Autodesk Inventor part; units mm, degrees
ref_plane "YZ Plane" through (0, 0, 0) normal (1, 0, 0) x (0, 1, 0)
ref_plane "XZ Plane" through (0, 0, 0) normal (0, 1, 0) x (-1, 0, 0)
ref_plane "XY Plane" through (0, 0, 0) normal (0, 0, 1) x (1, 0, 0)
sketch "Sketch1" plane through (0, 0, 0) normal (0, 1, 0) x (-1, 0, 0)
  circle A0 centre (18.5, 28) radius 23.85
  circle A1 centre (37, -23.25) radius 13.85
  circle A2 centre (-35, -38.75) radius 13.85
  circle A3 centre (-30.9, 25.8) radius 13.85
  circle A4 centre (0, -23.25) radius 13.85
  line L0 (56.25, 58.25) -> (-56.25, 58.25)
  line L1 (-56.25, -58.25) -> (56.25, -58.25)
  line L2 (0, -105.9299) -> (0, 123.2086) construction
  line L3 (-76.4777, -38.75) -> (-5.35, -38.75) construction
  line L4 (-123.5447, -23.25) -> (82.5572, -23.25) construction
  line L5 (56.25, -58.25) -> (56.25, 58.25)
  line L6 (56.25, 58.25) -> (56.25, -58.25)
  line L7 (-56.25, 58.25) -> (-56.25, -58.25)
  line L8 (100.0459, 28) -> (-13.85, 28) construction
  line L9 (-9.7154, 25.8) -> (-68.4996, 25.8) construction
  line L10 (18.5, 82.6038) -> (18.5, -4.654) construction
  line L11 (-30.9, 82.6038) -> (-30.9, 8.6393) construction
  point P0 (0, 0)
  point P1 (0, 0)
  dimension "d0" = 47.7
  dimension "d1" = 27.7
  dimension "d2" = 27.7
  dimension "d3" = 27.7
  dimension "d4" = 27.7
  dimension "d7" = 37
  dimension "d9" = 30.9
  dimension "d10" = 19.5
  dimension "d11" = 35
  dimension "d12" = 35
  dimension "d13" = 25.8
  dimension "d14" = 28
  dimension "d15" = 56.25
  dimension "d16" = 58.25
  dimension "d17" = 116.5
  dimension "d18" = 112.5
  dimension "d19" = 18.5
  dimension "d20" = 32.45
extrude "Extrusion1" add sketch "Sketch1" along normal blind 5
sketch "Sketch2" plane through (0, 5, 0) normal (0, 1, 0) x (1, 0, 0)
  line L0 (-56.25, 58.25) -> (-56.25, -58.25)
  line L1 (-56.25, -58.25) -> (56.25, -58.25)
  line L2 (56.25, -58.25) -> (56.25, 58.25)
  line L3 (56.25, 58.25) -> (-56.25, 58.25)
  circle A0 centre (0, 23.25) radius 13.85
  circle A1 centre (30.9, -25.8) radius 13.85
  circle A2 centre (35, 38.75) radius 13.85
  circle A3 centre (-37, 23.25) radius 13.85
  circle A4 centre (-18.5, -28) radius 23.85
  line L4 (-56.25, 58.25) -> (-56.25, -58.25)
  line L5 (-56.25, 23.25) -> (15.75, 23.25)
  line L6 (19.75, 38.75) -> (56.25, 38.75)
  line L7 (56.25, -58.25) -> (56.25, 58.25)
  line L8 (17.75, 25.25) -> (17.75, 36.75)
  arc A5 (15.75, 23.25) -> (17.75, 25.25) centre (15.75, 25.25) ccw
  arc A6 (19.75, 38.75) -> (17.75, 36.75) centre (19.75, 36.75) ccw
  point P0 (0, 0)
  point P1 (17.75, 23.25)
  point P2 (17.75, 38.75)
  point P3 (-50.85, 23.25)
  point P4 (-23.15, 23.25)
  point P5 (-13.85, 23.25)
  point P6 (13.85, 23.25)
  point P7 (21.15, 38.75)
  point P8 (48.85, 38.75)
  dimension "d23" = 74
  dimension "d25" = 38.5
  dimension "d26" = 2
  dimension "d27" = 35
  dimension "d28" = 19.5
sketch "Sketch3" plane through (0, 5, 0) normal (0, 1, 0) x (1, 0, 0)
  line L0 (-56.25, -28) -> (8.75, -28)
  line L1 (12.3221, -25.8) -> (56.25, -25.8)
  line L2 (-56.25, 58.25) -> (-56.25, -58.25)
  line L3 (-56.25, -58.25) -> (56.25, -58.25)
  line L4 (56.25, -58.25) -> (56.25, 58.25)
  line L5 (56.25, 58.25) -> (-56.25, 58.25)
  circle A0 centre (0, 23.25) radius 13.85
  circle A1 centre (30.9, -25.8) radius 13.85
  circle A2 centre (35, 38.75) radius 13.85
  circle A3 centre (-37, 23.25) radius 13.85
  circle A4 centre (-18.5, -28) radius 23.85
  line L6 (56.25, -58.25) -> (56.25, 58.25)
  line L7 (-56.25, 58.25) -> (-56.25, -58.25)
  line L8 (10.75, -26) -> (10.75, -25.8)
  arc A5 (8.75, -28) -> (10.5361, -26.9) centre (8.75, -26) ccw
  arc A6 (12.3221, -25.8) -> (10.5361, -26.9) centre (12.3221, -27.8) ccw
  point P0 (0, 0)
  point P1 (10.75, -28)
  point P2 (-42.35, -28)
  point P3 (5.35, -28)
  point P4 (17.05, -25.8)
  point P5 (44.75, -25.8)
  dimension "d29" = 67
  dimension "d30" = 2
extrude "Extrusion2" cut sketch "Sketch2" against normal through all contours L3 L2 L6 A2 A6 L8 A5 L5 A0 A3 L0
extrude "Extrusion3" cut sketch "Sketch3" against normal blind 10 contours A4 L0 L2 L5 L4 L1 A1 A6 A5
sketch "Sketch4" plane through (0, 5, 0) normal (0, 1, 0) x (1, 0, 0)
  line L0 (-56.25, -58.25) -> (56.25, -58.25)
  line L1 (56.25, -58.25) -> (28.75, -58.25)
  line L2 (28.75, -58.25) -> (28.75, -50.25)
  line L3 (30.75, -48.25) -> (56.25, -48.25)
  line L4 (56.25, -48.25) -> (56.25, -58.25)
  arc A0 (30.75, -48.25) -> (28.75, -50.25) centre (30.75, -50.25) ccw
  point P0 (0, 0)
  point P1 (28.75, -48.25)
  dimension "d35" = 27.5
  dimension "d36" = 10
  dimension "d37" = 2
extrude "Extrusion4" cut sketch "Sketch4" against normal through all
sketch "Sketch5" plane through (0, 5, 0) normal (0, 1, 0) x (1, 0, 0)
  line L0 (-56.25, -28) -> (-56.25, -58.25)
  line L1 (56.25, -48.25) -> (56.25, -25.8)
  line L2 (-56.25, -58.25) -> (28.75, -58.25)
  line L3 (-51.25, -39.75) -> (-40.25, -39.75)
  line L4 (-40.25, -39.75) -> (-40.25, -46.75)
  line L5 (-40.25, -46.75) -> (-51.25, -46.75)
  line L6 (-51.25, -46.75) -> (-51.25, -39.75)
  line L7 (40.25, -39.75) -> (51.25, -39.75)
  line L8 (51.25, -39.75) -> (51.25, -46.75)
  line L9 (51.25, -46.75) -> (40.25, -46.75)
  line L10 (40.25, -46.75) -> (40.25, -39.75)
  point P0 (0, 0)
  point P1 (-45.25, -43.25)
  point P2 (45.25, -43.25)
  dimension "d40" = 11
  dimension "d41" = 11
  dimension "d42" = 15
  dimension "d43" = 15
  dimension "d44" = 11
  dimension "d45" = 7
  dimension "d46" = 11
  dimension "d47" = 7
  dimension "d48" = 6
  dimension "d49" = 3.5
  dimension "d50" = 6
  dimension "d51" = 3.5
hole "Hole1" at (-45.25, 5, 43.25) at (45.25, 5, 43.25) direction (0, -1, 0) diameter 5.1 end through all
fillet "Fillet1" radius 4 2 edges at (-56.25, 2.5, 28) (56.25, 2.5, 25.8)
fillet "Fillet2" radius 2 3 edges at (-56.25, 2.5, 58.25) (28.75, 2.5, 58.25) (56.25, 2.5, 48.25)
properties part number "Top Bottle Front"
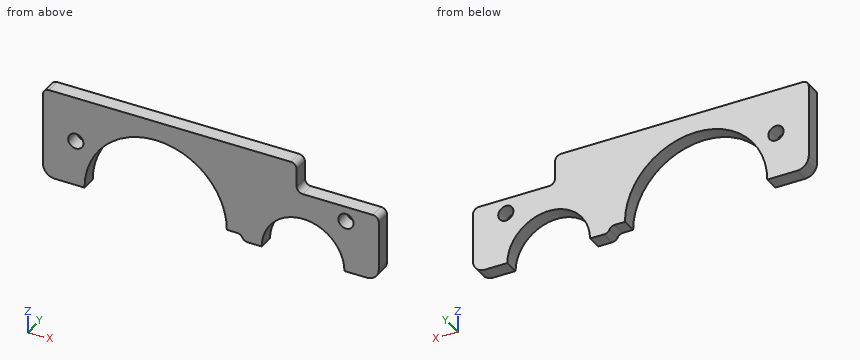
Here's how the part is built. I have some questions about the finished solid (model axes, mm). Round coordinates to 2 decimals unless told otherwise and drop trailing zeros. Order: outer loops, then holes, each group sorted by start corner. A loop starts at its lowest first (then second) coordinate and runs counter-clockwise, first axis right, second up. Notation, with made-up numbers: (-29, 25.25) -> (3, 25.25) arc R14 ccw to (3, 35.25) -> close; hole circle Ø1 at (10.25, 41.5). An arc over 180 degrees is marked (long way). Return JSON: item names as keys, results as strings.
Q1. If we section it at D-D on x = 2.5: List the corners of the cut face in (y, z) for me, plus the area to 3 significant figures.
Filled sheet:
{"outline": "(0, 39.31) -> (5, 39.31) -> (5, 58.25) -> (0, 58.25) -> close", "area": "94.7 mm^2"}
Q2. If we section it at A-A on y = 3.1: List the corners of the cut face in (x, z) for me, plus the area to 3 significant figures.
Filled sheet:
{"outline": "(-56.25, 32) arc R4 ccw to (-52.25, 28) -> (-42.35, 28) arc R23.85 cw to (5.35, 28) -> (8.75, 28) arc R2 cw to (10.54, 26.9) arc R2 ccw to (12.32, 25.8) -> (17.05, 25.8) arc R13.85 cw to (44.75, 25.8) -> (52.25, 25.8) arc R4 ccw to (56.25, 29.8) -> (56.25, 46.25) arc R2 ccw to (54.25, 48.25) -> (30.75, 48.25) arc R2 cw to (28.75, 50.25) -> (28.75, 56.25) arc R2 ccw to (26.75, 58.25) -> (-54.25, 58.25) arc R2 ccw to (-56.25, 56.25) -> close; hole circle Ø5.1 at (-45.25, 43.25); hole circle Ø5.1 at (45.25, 43.25)", "area": "1,980 mm^2"}
Q3. If we section it at C-C on x = -18.5: List the corners of the cut face in (y, z) for me.
Filled sheet:
{"outline": "(0, 51.85) -> (5, 51.85) -> (5, 58.25) -> (0, 58.25) -> close"}
Q4. For pin 1 Ø1 at (x, y) = (6.5, 2) entering from -Z; pin 2 Ø1.5 at (x, y) = (39.5, 1.5) entering from +Z; pin 3 Ø2 at (x, y) = (38, 4.5) entering from -Z, each with a flat end and sliding along its axis, tell me the tip position at first contact or that it passes through.
Filled sheet:
{"pin 1": "stops at z = 28", "pin 2": "stops at z = 48.25", "pin 3": "stops at z = 37.03"}
Q5. I need wall thicknesses on line 1 along Z through (x, y) = (45.25, 2.35); line 2 along Z through (x, y) = (-45.25, 3.55); line 3 along X through (y, z) = (1.95, 43.25). Which ranges of each line are inside material? Lowest first, please. Write a range as from..to.
Filled sheet:
{"line 1": "z = 25.8..40.7, 45.8..48.25", "line 2": "z = 28..40.7, 45.8..58.25", "line 3": "x = -56.25..-47.8, -42.7..-36.84, -0.16..42.7, 47.8..56.25"}
Q6. If we section it at B-B on z = 37: List the corners of the cut face in (x, y) for me.
Filled sheet:
{"outline": "(-56.25, 0) -> (-40.59, 0) -> (-40.59, 5) -> (-56.25, 5) -> close; (3.59, 0) -> (22.75, 0) -> (22.75, 5) -> (3.59, 5) -> close; (39.05, 0) -> (56.25, 0) -> (56.25, 5) -> (39.05, 5) -> close"}
